Autodesk Inventor part; units mm, degrees
ref_plane "YZ Plane" through (0, 0, 0) normal (1, 0, 0) x (0, 1, 0)
ref_plane "XZ Plane" through (0, 0, 0) normal (0, 1, 0) x (-1, 0, 0)
ref_plane "XY Plane" through (0, 0, 0) normal (0, 0, 1) x (1, 0, 0)
sketch "Sketch1" plane through (0, 0, 0) normal (0, 0, 1) x (1, 0, 0)
  line L0 (130.175, 215.9) -> (200.025, 215.9)
  line L1 (130.175, 215.9) -> (25.4, 0)
  line L2 (200.025, 215.9) -> (304.8, 0)
  line L3 (306.7883, 3.175) -> (202.0133, 219.075)
  line L4 (202.0133, 219.075) -> (128.1867, 219.075)
  line L5 (128.1867, 219.075) -> (23.4117, 3.175)
  line L6 (25.4, 0) -> (50.1039, 0)
  line L7 (50.1039, 0) -> (154.1085, 214.3125)
  line L8 (172.5624, 214.3125) -> (276.567, 0)
  line L9 (276.567, 0) -> (304.8, 0)
  line L10 (129.4046, 214.3125) -> (154.1085, 214.3125)
  line L11 (172.5624, 214.3125) -> (200.7954, 214.3125)
  line L12 (50.1039, 0) -> (276.567, 0) construction
  line L13 (25.4, 0) -> (0, 0)
  line L14 (0, 0) -> (0, 3.175)
  line L15 (0, 3.175) -> (23.4117, 3.175)
  line L16 (304.8, 0) -> (330.2, 0)
  line L17 (330.2, 0) -> (330.2, 3.175)
  line L18 (330.2, 3.175) -> (306.7883, 3.175)
  dimension "d1" = 69.85
  dimension "d5" = 3.175
  dimension "d34" = 22.225
  dimension "d35" = 25.4
  dimension "d37" = 1.5875
  dimension "d41" = 3.175
  dimension "d43" = 219.075
  dimension "d44" = 3.175
  dimension "d45" = 64.113
  dimension "d46" = 64.113
  dimension "d47" = 3.175
  dimension "d48" = 25.4
  dimension "d49" = 25.4
  dimension "d50" = 330.2
extrude "Extrusion1" add sketch "Sketch1" along normal blind 25.4 contours L1 L13 L14 L15 L5 L4 L3 L18 L17 L16 L2 L0
extrude "Extrusion2" add sketch "Sketch1" along normal blind 3.175
fillet "Fillet1" radius 0.7937 6 edges at (130.175, 215.9, 12.7) (200.025, 215.9, 12.7) (200.7954, 214.3125, 1.5875) (129.4046, 214.3125, 1.5875) (23.4117, 3.175, 12.7) (306.7883, 3.175, 12.7)
fillet "Fillet2" radius 3.175 4 edges at (128.1867, 219.075, 12.7) (202.0133, 219.075, 12.7) (25.4, 0, 14.2875) (304.8, 0, 14.2875)
equation "\"d5\" = d4"
equation "\"d37\" = d36"
equation "\"d44\" = d41"
equation "\"d45\" = d46"
equation "\"d47\" = d41"
equation "\"d49\" = d48"
equation "\"d36\" = 0.5 * d5"
properties part number "8 ball lift frame"
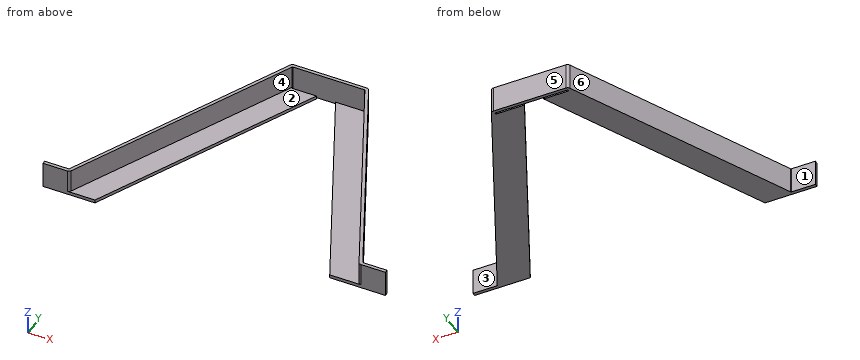
Check sheet for the modelled part. Datum: model origin and axes. Units: mm. Face numbers are marked on the shaded views. A direction names the side the tool comes from. Give positions to 0.01 mm unless a question says otherwise; leave off trailing zeros. Order: outer loops, then holes, each group sorted by start corner. A loop starts at its lowest first (then second) coordinate and runs counter-clockwise, first axis right, second up. Notation, with made-up numbers: M 25,76.5 L 68,76.5 A24 cw 68,101.5 Z; hole C -37.5,82.5 d1. An arc over 180 degrees is marked long. Answer in a Markdown table with one row per item. Add a question column.
Q1. Sectioned sample at B-B, the plane y = 48. Record the boundary of the cut face in (x, z) (3 decimals), and give its area (3 significant figures).
Q2. Sectioned sample at C-C, the plane x = 176. Record the boundary of the cut face in (y, z) (1 decimal), and give its area (3 significant figures).
Q3. Release check for a two-part mould opening along X. For the marked faces 4, 5 and 6 record: released by +X, released by -X, zero draft, split by the parting line, or undercut.
Q4. Sectioned sample at D-D, the plane x = 256.5. Record the boundary of the cut face in (y, z) (3 decimals).
Q5. Sectioned sample at A-A, the plane z = 21.25. Record the boundary of the cut face in (x, y) (3 decimals), and give its area (3 significant figures).
Q6. Gauge pin test, flat ends, axial feed: pin 1 Ø8 at (x, z) = (295, 18.5) entering from +Y; pin 2 Ø2 at (y, z) = (134.5, 17.5) entering from +X; pin 3 Ø10 at (y, z) = (59, 20.5) entering from -X. Record the tip position at first contact, or that the pin passes through.
Q7. Thickness scan on L1, parallel to Y at x = 136, z = 13 (3 decimals); L2, parallel to X at y = 52, z = 9.25; L3, parallel to X at y = 177, z = 16.25. Record the ranges inside material, lowest first.
Q8. Access from +Z, -Z, +X, -X, +Y, -Y to the whole of each face (thin tool, end or side, straight path). Record for the marked faces 1, 2 and 3.
Verdict:
| question | item | result |
|---|---|---|
| 1 | outline | M 45.165,0 L 73.398,0 L 73.398,3.175 L 48.694,3.175 L 48.694,25.4 L 45.165,25.4 Z; M 253.273,0 L 285.035,0 L 285.035,25.4 L 281.506,25.4 L 281.506,3.175 L 253.273,3.175 Z |
| 1 | area | 347 mm² |
| 2 | outline | M 207.2,0 L 214.3,0 L 214.3,3.2 L 207.2,3.2 Z; M 215.9,0 L 219.1,0 L 219.1,25.4 L 215.9,25.4 Z |
| 2 | area | 103 mm² |
| 3 | face 4 | undercut |
| 3 | face 5 | zero draft |
| 3 | face 6 | released by -X |
| 4 | outline | M 41.35,0 L 106.799,0 L 106.799,25.4 L 99.527,25.4 L 99.527,3.175 L 41.35,3.175 Z |
| 5 | outline | M 0,0 L 23.412,0 A3.175 ccw 26.268,1.789 L 129.958,215.453 A0.794 cw 130.672,215.9 L 199.528,215.9 A0.794 cw 200.242,215.453 L 303.932,1.789 A3.175 ccw 306.788,0 L 330.2,0 L 330.2,3.175 L 307.285,3.175 A0.794 cw 306.571,3.622 L 202.881,217.286 A3.175 ccw 200.025,219.075 L 130.175,219.075 A3.175 ccw 127.319,217.286 L 23.629,3.622 A0.794 cw 22.915,3.175 L 0,3.175 Z |
| 5 | area | 1,900 mm² |
| 6 | pin 1 | y = 35.71 |
| 6 | pin 2 | x = 243.54 |
| 6 | pin 3 | x = 48.08 |
| 7 | L1 | 215.9 to 219.075 |
| 7 | L2 | 47.11 to 50.64, 279.56 to 283.09 |
| 7 | L3 | 107.77 to 111.3, 218.9 to 222.43 |
| 8 | face 1 | +Z, -Z, -X, +Y |
| 8 | face 2 | +Z, -Y |
| 8 | face 3 | +Z, -Z, +X, +Y |
